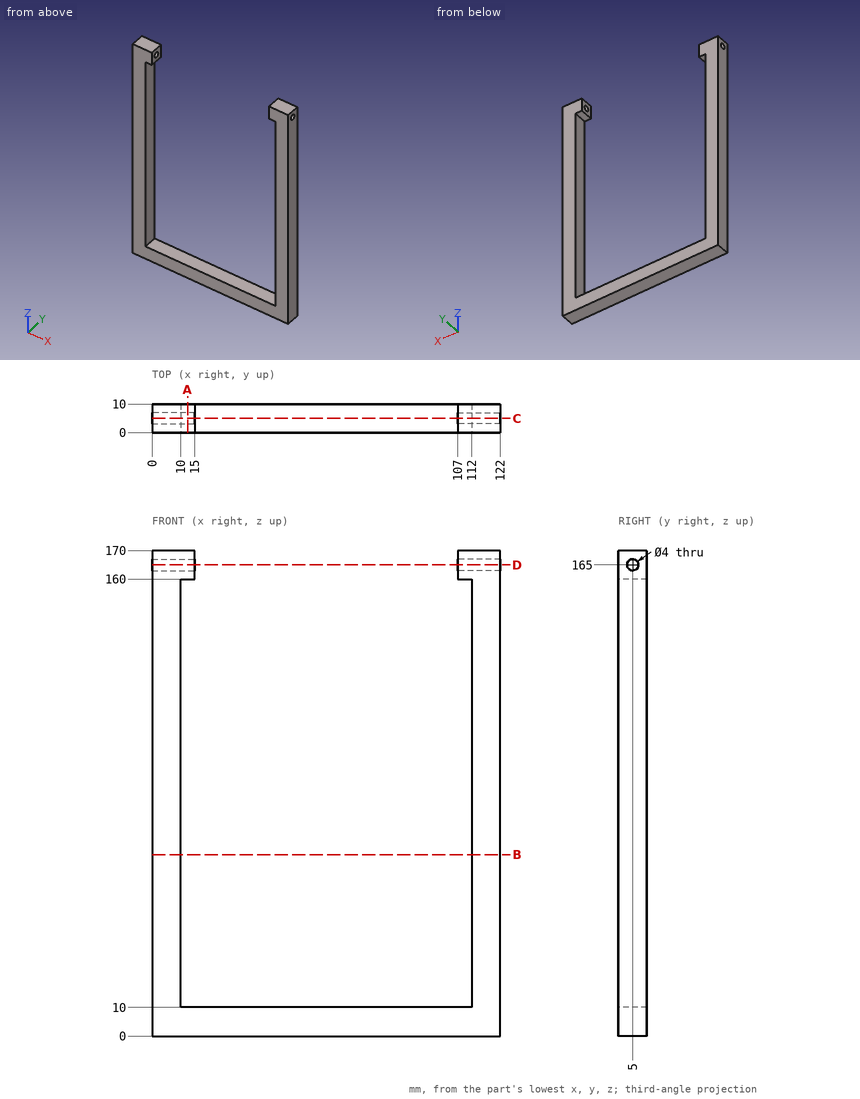
Part print with two shaded views. Sizes in mm from the minimum x, y, z corner. Round coordinates to 2 decimals unless told otherwise and drop trailing zeros. Write each loop counter-clockwise with the first axis right and the second up, starting at its lowest first coordinate (ties: lowest second). Pieces come first, ordered by that corner, then holes. Notation, with made-up numbers: M 87.25,10.5 L 101.25,10.5 A25 cw 101.25,24.5 Z; hole C 29,28 d4. An arc over 180 degrees is marked long. Answer as CSV lines item,"result". Start each with the question number.
1) Band-saw the part on A-A (x = 12.5). List the corners of the cut face in (y, z).
2) Band-saw the part on C-C (y = 5). List the corners of the cut face in (x, z).
3) Band-saw the part on B-B (z = 63.5). List the corners of the cut face in (x, y).
4) Drill centre lines: L1, parallel to X at y = 2.5, z = 49; L2, parallel to Z at x = 113, y = 5; L3, parallel to Y at x = 10.5, z = 165. Where is each one in solid material? Low to high.
5) Band-saw the part on D-D (z = 165). List the corners of the cut face in (x, y).
6) Drop flat-ended pins along their axis: pin 1 (3 mm diameter, centred on x = 20.5, y = 7.5, fed in from +Z); pin 2 (3 mm diameter, centred on y = 5, z = 165, fed in from -X). Give the stop position or say it passes through.
Worked out:
1,outline,"M 0,0 L 10,0 L 10,10 L 0,10 Z; M 0,160 L 10,160 L 10,170 L 0,170 Z; hole C 5,165 d4"
2,outline,"M 0,0 L 122,0 L 122,163 L 107,163 L 107,160 L 112,160 L 112,10 L 10,10 L 10,160 L 15,160 L 15,163 L 0,163 Z; M 0,167 L 15,167 L 15,170 L 0,170 Z; M 107,167 L 122,167 L 122,170 L 107,170 Z"
3,outline,"M 0,0 L 10,0 L 10,10 L 0,10 Z; M 112,0 L 122,0 L 122,10 L 112,10 Z"
4,L1,"0 to 10, 112 to 122"
4,L2,"0 to 163, 167 to 170"
4,L3,"0 to 3, 7 to 10"
5,outline,"M 0,0 L 15,0 L 15,3 L 0,3 Z; M 0,7 L 15,7 L 15,10 L 0,10 Z; M 107,0 L 122,0 L 122,3 L 107,3 Z; M 107,7 L 122,7 L 122,10 L 107,10 Z"
6,pin 1,"z = 10"
6,pin 2,"through"
